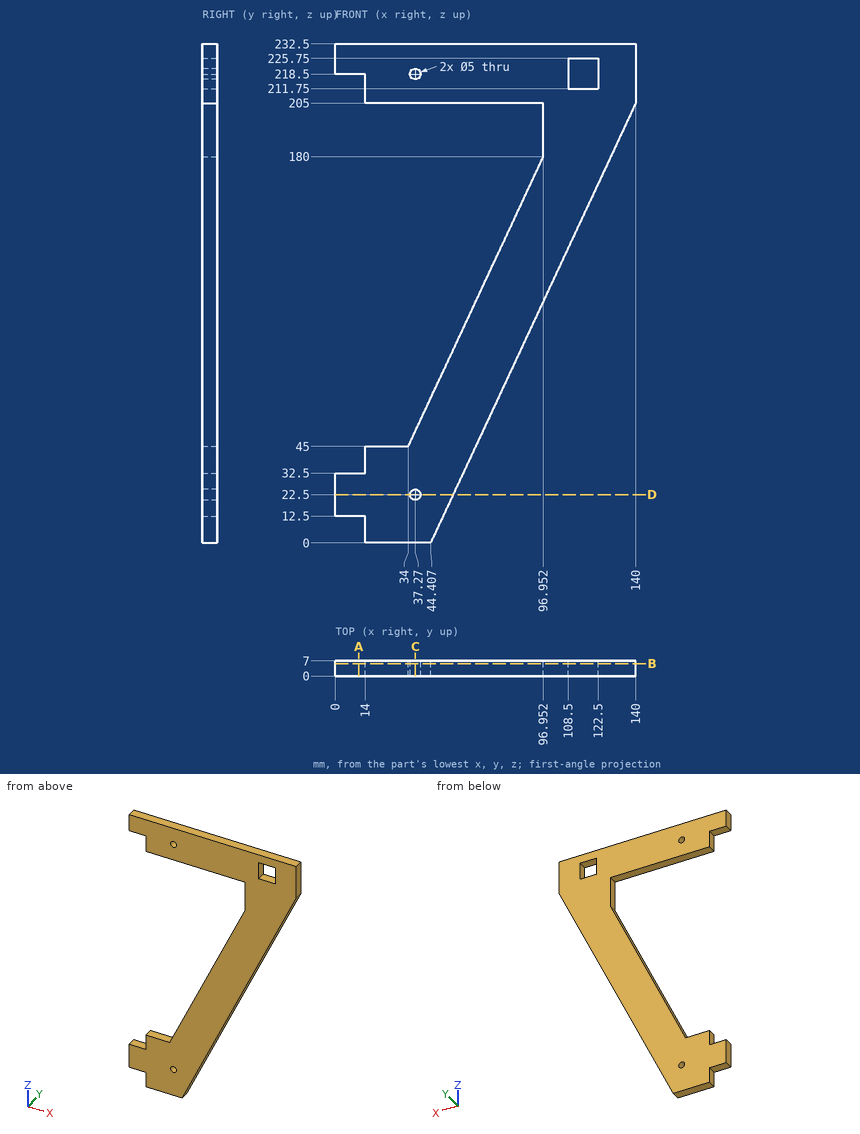
Verification items for this drawing (mm, ordinates from the low corner). Coordinates: 2 decimals unless noted, no trailing zeros. Write each loop counter-clockwise with the first axis right and the second up, starting at its lowest first coordinate (ties: lowest second). Pieces come first, ordered by that corner, then holes. Notation, with made-up numbers: M 51.25,62 L 93.25,62 A28 ccw 93.25,95 Z; hole C -8,-36.75 d9. An arc over 180 degrees is marked long. Answer as a JSON object with one key per item and string values. Group by question number.
(1) Cross-section at C-C, the plane x = 37.27. Record the cut outline in (y, z).
(2) Cross-section at B-B, the plane y = 5.75. Record the cut outline in (x, z).
(3) Material ranges on line 1 (Z direction, x = 37.27, y = 5.75) (1 decimal); line 2 (Z direction, x = 19.5, y = 4.5); line 3 (Z direction, x = 12.5, y = 3.75), recorded low to high.
(4) Cross-section at D-D, the plane z = 22.5. Record the cut outline in (x, y).
(5) Gauge pin test, flat ends, axial feed: pin 1 (1.5 mm diameter, centred on x = 59.5, y = 4.5, fed in from -Z); pin 2 (4 mm diameter, centred on y = 6, z = 106, fed in from -X); pin 3 (1 mm diameter, centred on y = 1.5, z = 139.5, fed in from -X). Record the tip position at first contact, or that the pin passes through.
(6) Cross-section at A-A, the plane x = 11. Record the cut outline in (y, z).
Reply:
{
 "1": {"outline": "M 0,0 L 7,0 L 7,20 L 0,20 Z; M 0,25 L 7,25 L 7,52.01 L 0,52.01 Z; M 0,205 L 7,205 L 7,216 L 0,216 Z; M 0,221 L 7,221 L 7,232.5 L 0,232.5 Z"},
 "2": {"outline": "M 0,12.5 L 14,12.5 L 14,0 L 44.41,0 L 140,205 L 140,232.5 L 0,232.5 L 0,218.5 L 14,218.5 L 14,205 L 96.95,205 L 96.95,180 L 34,45 L 14,45 L 14,32.5 L 0,32.5 Z; hole C 37.27,22.5 d5; hole C 37.27,218.5 d5; hole M 108.5,211.75 L 122.5,211.75 L 122.5,225.75 L 108.5,225.75 Z"},
 "3": {"line 1": "0 to 20, 25 to 52, 205 to 216, 221 to 232.5", "line 2": "0 to 45, 205 to 232.5", "line 3": "12.5 to 32.5, 218.5 to 232.5"},
 "4": {"outline": "M 0,0 L 34.77,0 L 34.77,7 L 0,7 Z; M 39.77,0 L 54.9,0 L 54.9,7 L 39.77,7 Z"},
 "5": {"pin 1": "z = 30.76", "pin 2": "x = 61.51", "pin 3": "x = 77.83"},
 "6": {"outline": "M 0,12.5 L 7,12.5 L 7,32.5 L 0,32.5 Z; M 0,218.5 L 7,218.5 L 7,232.5 L 0,232.5 Z"}
}
